Design review of the part built by this model. Coordinates are the model's own, in mm. A direction names the side the tool comes from. Give positions to 0.01 mm unless a question says otherwise; leave off trailing zeros. Loops run counter-clockwise (first coordinate to the right, second up) from the corner with the lowest first, then second, coordinate; pieces in that order, holes last. Notation, with made-up numbers: (84, 69.25) -> (141, 69.25) arc R17 cw to (141, 83.25) -> close; hole circle Ø2 at (52.5, 32). An arc over 180 degrees is marked (long way). Use a Markdown table: item, result. Add a question column.
1. Draft analysis for pull direction X (two halves, no side actions). For faces 1 (the flat face through (3, -13, 0)), 2 (the flat face through (21.277, -12.878, 12.908)), 3 (the flat face through (13.88, -12.88, 18.57)), state which applies: pulls with the +X half, pulls with the -X half, needs draft (parallel to the pull), parting line crosses it, or undercut.
2. Add section A-A (y = -19.25). State the section outline as (x, z) points, and give its area (3 significant figures).
3. To check wall thickness, follow line 1 (Z direction, x = 12.5, y = -21.5); line 2 (X direction, y = -18.25, z = 5.5); line 3 (Z direction, x = 11.75, y = -18.5). State the ranges of each line that lie inside material, in increasing order.
4. Add section D-D (y = -2). Count the separate pieces of the cut face and the enclosed holes in it, and give its area (3 significant figures).
5. For faces 4 (the flat face through (13, 0, 13)), 5 (the flat face through (7.475, -12.878, 4.419)), 6 (the flat face through (10.77, -12.88, 18.71)), list the 3-axis set-ups (+Z, -Z, +X, -X, +Y, -Y) from which the entire face can be reached by the end or side of a thin tool; tool diameter is ignored.
6. For pin 1 Ø3 at (x, z) = (12.5, 17) entering from +Y; pin 2 Ø10 at (y, z) = (-12, 25.5) entering from +X; pin 3 Ø6 at (y, z) = (-14.5, 27.5) entering from +X; pin 4 Ø4 at (x, y) = (9.5, -20.5) entering from +Z, all flat-tipped, find the tip position at first contact; note any pin that passes through.
7. Add section C-C (x = 13). State the section outline as (y, z) points (3 decimals).
8. Add section B-B (z = 18.5). State the section outline as (x, y) points, and give its area (3 significant figures).
```python
from build123d import *

# Parameters (mm, degrees)
F1_DEPTH = 25.4
F3_DEPTH = 25.4
F5_R     = 1.5875


with BuildPart() as f1:
    # F0 (on Front) → F1 (new body)
    with BuildSketch(Plane.XZ):
        Polygon((25.399335, 25.4), (0, 25.583795), (0, 0), (25.399335, 0), align=None)
    extrude(amount=F1_DEPTH)

    # F2 (on face) → F3 (cut)
    with BuildSketch(Plane.XZ.offset(25.4)):
        Polygon((0, 0), (7.961136, 25.526187), (0, 25.583795), align=None)
        Polygon((9.200284, 8.716307), (5.701287, 0), (18.071296, 0), (15.525086, 8.660929), align=None)
        Polygon((25.399335, 25.4), (17.26905, 25.458833), (25.399335, 0), align=None)
        Polygon((9.184068, 15.181166), (15.411005, 15.101977), (12.307478, 22.137856), align=None)
    extrude(amount=-F3_DEPTH, mode=Mode.SUBTRACT)

    # F5 (on offset) → F6 (revolve)
    with BuildSketch(Plane.XZ.offset(6.35)):
        with Locations((12.7, 25.4)):
            Circle(F5_R)
    revolve(axis=Axis((14.252264, -6.35, 28.575), (1, 0, 0)))


solid = f1.part
```
Taken from the geometry:
| question | item | result |
|---|---|---|
| 1 | face 1 | needs draft |
| 1 | face 2 | pulls with the +X half |
| 1 | face 3 | undercut |
| 2 | outline | (0, 0) -> (5.7, 0) -> (9.2, 8.72) -> (15.53, 8.66) -> (18.07, 0) -> (25.4, 0) -> (17.27, 25.46) -> (7.96, 25.53) -> close; hole (9.18, 15.18) -> (15.41, 15.1) -> (12.31, 22.14) -> close |
| 2 | area | 339 mm^2 |
| 3 | line 1 | z = 8.69 to 15.14, 21.7 to 25.49 |
| 3 | line 2 | x = 1.72 to 7.91, 16.45 to 23.64 |
| 3 | line 3 | z = 8.69 to 15.15, 20.9 to 25.5 |
| 4 | separate pieces | 2 |
| 4 | enclosed holes | 1 |
| 4 | area | 346 mm^2 |
| 5 | face 4 | +Z, -Z, +X, -X, +Y |
| 5 | face 5 | -Z, +Y, -Y |
| 5 | face 6 | +Y, -Y |
| 6 | pin 1 | passes through |
| 6 | pin 2 | stops at x = 18.85 |
| 6 | pin 3 | stops at x = 17.58 |
| 6 | pin 4 | stops at z = 25.53 |
| 7 | outline | (-25.4, 8.683) -> (0, 8.683) -> (0, 15.133) -> (-25.4, 15.133) -> close; (-25.4, 20.568) -> (0, 20.568) -> (0, 25.49) -> (-2.76, 25.49) arc R4.734 ccw (long way) to (-9.94, 25.49) -> (-25.4, 25.49) -> close; hole circle Ø3.232 at (-6.35, 28.575) |
| 8 | outline | (5.77, -25.4) -> (10.67, -25.4) -> (10.67, 0) -> (5.77, 0) -> close; (13.91, -25.4) -> (19.49, -25.4) -> (19.49, 0) -> (13.91, 0) -> close |
| 8 | area | 266 mm^2 |
